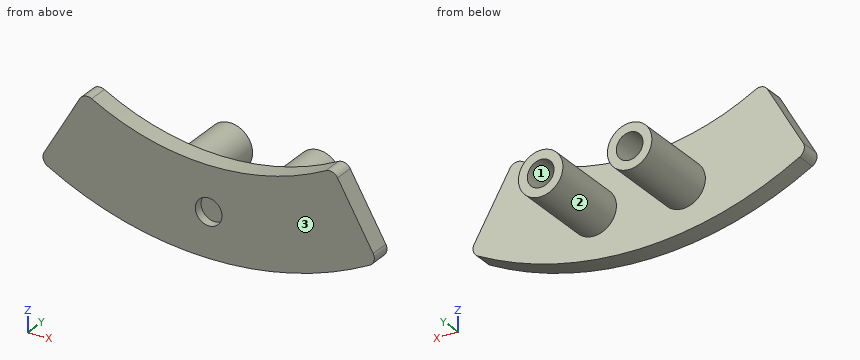
```python
from build123d import *

# Parameters (mm, degrees)
BOSS_EXTRUDE1_DEPTH = 2.2
SKETCH2_R           = 2.5
BOSS_EXTRUDE2_DEPTH = 9.3
SKETCH5_R           = 1.5
CUT_EXTRUDE1_DEPTH  = 3.5
SKETCH6_R           = 1.5
CUT_EXTRUDE2_DEPTH  = 1
FILLET1_R           = 1


with BuildPart() as part:
    # Sketch1 → Boss-Extrude1 (new body)
    with BuildSketch(Plane(origin=(0, 0, 0), x_dir=(1, 0, 0), z_dir=(0, 1, 0))):
        with BuildLine():
            Line((-19, 32.908965344), (-14, 24.248711306))
            ThreePointArc((-14, 24.248711306), (0, 28), (14, 24.248711306))
            Line((14, 24.248711306), (19, 32.908965344))
            ThreePointArc((19, 32.908965344), (0, 38), (-19, 32.908965344))
        make_face()
    extrude(amount=BOSS_EXTRUDE1_DEPTH)

    # Sketch2 → Boss-Extrude2 (add)
    with BuildSketch(Plane(origin=(0, 2.2, 0), x_dir=(1, 0, 0), z_dir=(0, 1, 0))):
        with Locations(Location((-5, 32.619012861, 0), (0, 0, 90))):
            Circle(SKETCH2_R)
        with Locations(Location((5, 32.619012861, 0), (0, 0, 90))):
            Circle(SKETCH2_R)
    extrude(amount=BOSS_EXTRUDE2_DEPTH)

    # Sketch5 → Cut-Extrude1 (cut)
    with BuildSketch(Plane(origin=(0, 11.5, 0), x_dir=(1, 0, 0), z_dir=(0, 1, 0))):
        with Locations(Location((-5, 32.619012861, 0), (0, 0, 270))):
            Circle(SKETCH5_R)
        with Locations(Location((5, 32.619012861, 0), (0, 0, 270))):
            Circle(SKETCH5_R)
    extrude(amount=-CUT_EXTRUDE1_DEPTH, mode=Mode.SUBTRACT)

    # Sketch6 → Cut-Extrude2 (cut)
    with BuildSketch(Plane.XZ):
        with Locations(Location((0, -33, 0), (0, 0, 270))):
            Circle(SKETCH6_R)
    extrude(amount=-CUT_EXTRUDE2_DEPTH, mode=Mode.SUBTRACT)

    # Fillet1
    fillet1_edges = [part.edges().sort_by_distance(p)[0] for p in [
        (19, 1.1, -32.908965344),
        (14, 1.1, -24.248711306),
        (-14, 1.1, -24.248711306),
        (-19, 1.1, -32.908965344),
    ]]
    fillet(fillet1_edges, radius=FILLET1_R)


solid = part.part
```
Read the model definition and answer for the solid it produces. Units are mm, in the model's axes. Face numbers are marked on the shaded views. Coordinates: 2 decimals unless noted, no trailing zeros. Write each loop counter-clockwise with the first axis right and the second up, starting at its lowest first coordinate (ties: lowest second). Pieces come first, ordered by that corner, then holes. Notation, with made-up numbers: (15, 32.25) - (50, 32.25) arc R22 cw to (50, 39.25) - close; hole circle Ø9 at (-32.5, -7). An arc over 180 degrees is marked (long way). Answer as a JSON object with one key per item and string values. Group by question number.
1. A cutting plane is placed at A-A (y = 9.25). Determine the outline of the cut face in (x, z), plus the area to 3 significant figures.
2. A cutting plane is placed at D-D (y = 5). Determine the outline of the cut face in (x, z), plus the area to 3 significant figures.
3. Consider L1, parallel to Y at x = -6, z = -36.5; L2, parallel to X at y = 4, z = -33.25; L3, parallel to Y at x = 0, z = -34.25. Determine where each line is inside the solid, lowest interval first. Write a range as [from, to].
4. A cutting plane is placed at C-C (x = 0). Determine the outline of the cut face in (y, z).
5. A cutting plane is placed at B-B (z = -26). Determine the outline of the cut face in (x, y), plus the area to 3 significant figures.
6. Each of these flat-tipped pins is pushed along its axis until it touches: P1, Ø5, axis at x = -14, y = 7, coming from the +Z side; P2, Ø0.9, axis at x = 4.5, z = -33.5, coming from the +Y side; P3, Ø2.5, axis at x = 0, z = -33, coming from the +Y side; P4, Ø6, axis at x = -8, y = 7.5, coming from the -Z side. Where does it stop, or does it pass through?
7. The mould has two halves that part along X. Classify the marked faces 1, 2 and 3: +X half, -X half, draft (parallel to the pull), parting line (faces both ways), or undercut.
Worked out:
{
 "1": {"outline": "circle Ø5 at (-5, -32.62); circle Ø5 at (5, -32.62); hole circle Ø3 at (-5, -32.62); hole circle Ø3 at (5, -32.62)", "area": "25.1 mm²"},
 "2": {"outline": "circle Ø5 at (-5, -32.62); circle Ø5 at (5, -32.62)", "area": "39.3 mm²"},
 "3": {"L1": "y = [0, 2.2]", "L2": "x = [-7.42, -2.58], [2.58, 7.42]", "L3": "y = [1, 2.2]"},
 "4": {"outline": "(0, -38) - (2.2, -38) - (2.2, -28) - (0, -28) - (0, -31.5) - (1, -31.5) - (1, -34.5) - (0, -34.5) - close"},
 "5": {"outline": "(-15.01, 0) - (-10.39, 0) - (-10.39, 2.2) - (-15.01, 2.2) - close; (10.39, 0) - (15.01, 0) - (15.01, 2.2) - (10.39, 2.2) - close", "area": "20.3 mm²"},
 "6": {"P1": "passes through", "P2": "stops at y = 8", "P3": "stops at y = 2.2", "P4": "stops at z = -35.12"},
 "7": {"face 1": "undercut", "face 2": "undercut", "face 3": "draft"}
}
